For this review, take the finished solid that the model builds, in its own axes (mm). A direction names the side the tool comes from. Coordinates: 2 decimals unless noted, no trailing zeros. Loops run counter-clockwise (first coordinate to the right, second up) from the corner with the lowest first, then second, coordinate; pieces in that order, holes last. Notation, with made-up numbers: (46, -7.5) - (65, -7.5) arc R19 cw to (65, 6.5) - close; hole circle Ø3 at (72.25, -22). An arc over 180 degrees is marked (long way). Use one line per item in the form item = value. Start each with the question number.
1. Add section C-C on x = 51. Give the boundary of the cut face in (y, z), and give its area (3 significant figures).
2. Add section D-D on z = 4.5. Give the boundary of the cut face in (x, y).
3. Add section B-B on y = 71.85. Give the boundary of the cut face in (x, z), and give its area (3 significant figures).
4. For pin 1 Ø4 at (x, y) = (-5, -4.15) entering from -Z, flat-tipped, find the tip position at first contact; note if it passes through.
5. Draft analysis for pull direction Y (two halves, no side actions). For faces 3 (the face through (-5.69, 70.52, 2.96)), 4 (the face through (52, 74, 0)), 5 (the face through (52, 78.85, 3)), state which applies: +Y half, -Y half, draft (parallel to the pull), parting line (faces both ways), or undercut.
6. Machinability: for faces 1 (the face through (52, -11.15, 3)), 2 (the face through (106, 33, 3)), which of the approach directions +Z, -Z, +X, -X, +Y, -Y give a long, thin tool a straight path to every point of the face, cutting with its end or side? Answer none if there is none.
7. To check wall thickness, follow probe 1 along X at (y, z) = (71.85, 3.55); probe 2 along Y at (x, z) = (-5, 2); probe 3 along X at (y, z) = (54, 5.5). State the ranges of each line that lie inside material, in increasing order.
8. Add section A-A on y = 54.5. Give the boundary of the cut face in (x, z), and give its area (3 significant figures).
```python
from build123d import *

# Parameters (mm, degrees)
SKETCH1_W             = 130
SKETCH1_H             = 90
SKETCH1_W_2           = 106
SKETCH1_H_2           = 67.7
BOSS_EXTRUDE1_DEPTH   = 6
F_3_0MM_DOWEL_HOLE1_D = 3


with BuildPart() as part:
    # Sketch1 → Boss-Extrude1 (new body)
    with BuildSketch(Plane.XY):
        with Locations((53, 33.85)):
            Rectangle(SKETCH1_W, SKETCH1_H)
        with Locations((53, 33.85)):
            Rectangle(SKETCH1_W_2, SKETCH1_H_2, mode=Mode.SUBTRACT)
    extrude(amount=BOSS_EXTRUDE1_DEPTH)

    # Ø3.0mm Dowel Hole1 (through all)
    with Locations(Plane.XY.offset(6)):
        with Locations((111, 71.85), (111, -4.15), (-5, -4.15), (-5, 71.85)):
            Hole(F_3_0MM_DOWEL_HOLE1_D / 2)


solid = part.part
```
Conclusion:
q1.outline = (-11.15, 0) - (0, 0) - (0, 6) - (-11.15, 6) - close; (67.7, 0) - (78.85, 0) - (78.85, 6) - (67.7, 6) - close
q1.area = 134 mm^2
q2.outline = (-12, -11.15) - (118, -11.15) - (118, 78.85) - (-12, 78.85) - close; hole circle Ø3 at (-5, -4.15); hole circle Ø3 at (-5, 71.85); hole (0, 0) - (106, 0) - (106, 67.7) - (0, 67.7) - close; hole circle Ø3 at (111, -4.15); hole circle Ø3 at (111, 71.85)
q3.outline = (-12, 0) - (-6.5, 0) - (-6.5, 6) - (-12, 6) - close; (-3.5, 0) - (109.5, 0) - (109.5, 6) - (-3.5, 6) - close; (112.5, 0) - (118, 0) - (118, 6) - (112.5, 6) - close
q3.area = 744 mm^2
q4.pin_1 = 0
q5.face_3 = undercut
q5.face_4 = draft
q5.face_5 = +Y half
q6.face_1 = +Z, -Z, +X, -X, -Y
q6.face_2 = +Z, -Z
q7.probe_1 = -12 to -6.5, -3.5 to 109.5, 112.5 to 118
q7.probe_2 = -11.15 to -5.65, -2.65 to 70.35, 73.35 to 78.85
q7.probe_3 = -12 to 0, 106 to 118
q8.outline = (-12, 0) - (0, 0) - (0, 6) - (-12, 6) - close; (106, 0) - (118, 0) - (118, 6) - (106, 6) - close
q8.area = 144 mm^2
